Could you check a few things on this drawing? It's one solid part, dimensions in mm from its lowest x, y, z. A direction names the side the tool comes from. Give positions to 0.01 mm unless a question says otherwise; leave off trailing zeros. Order: outer loops, then holes, each group sorted by start corner. A loop starts at its lowest first (then second) coordinate and runs counter-clockwise, first axis right, second up.
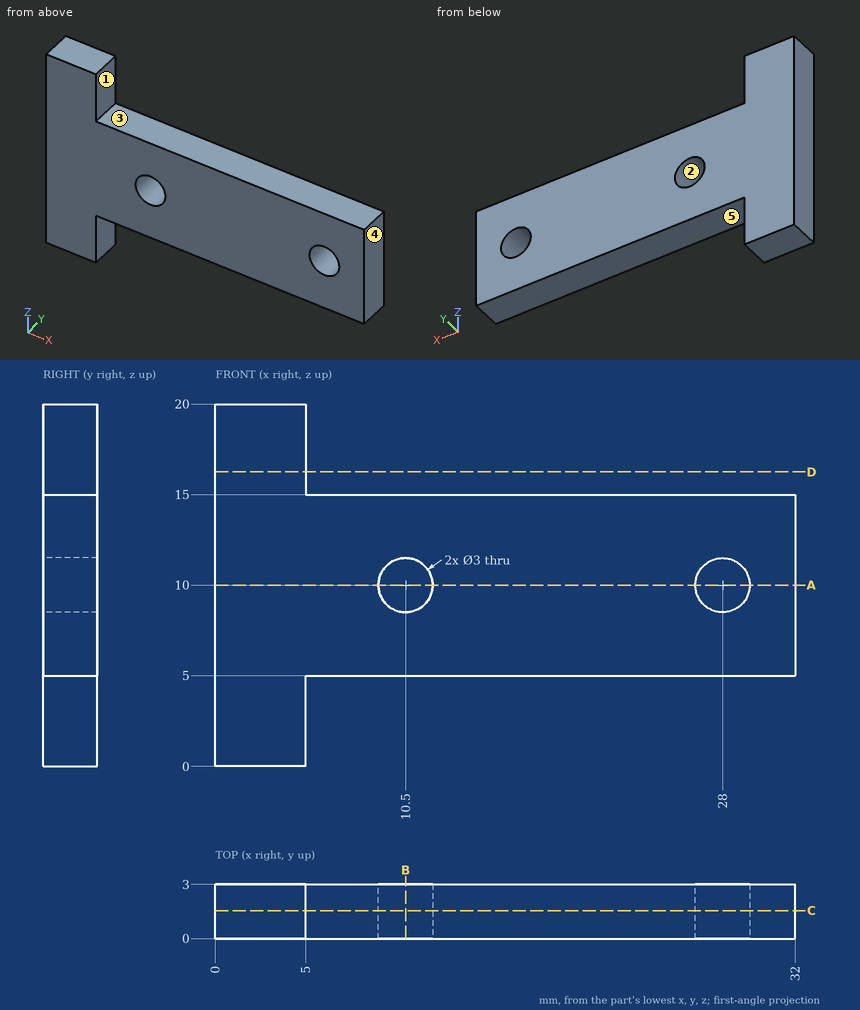
Q1. I'm going to push flat-ended pins straight in: P1, Ø1.5, axis at y = 1.5, z = 18.5, coming from the +X side; P2, Ø1.5, axis at x = 20, y = 1.5, coming from the -Z side. Where does each tip first touch, or does it pass through?
Filled sheet:
P1: stops at x = 5
P2: stops at z = 5
Q2. I need wall thicknesses on L1, parallel to Z at x = 28, y = 2.1; L2, parallel to Z at x = 25.5, y = 1.05; L3, parallel to X at y = 1.4, z = 9.75. Which ranges of each line are inside material? Lowest first, please.
Filled sheet:
L1: z = 5 to 8.5, 11.5 to 15
L2: z = 5 to 15
L3: x = 0 to 9.02, 11.98 to 26.52, 29.48 to 32
Q3. If we section it at C-C on y = 1.55: List the corners of the cut face in (x, z) for me, plus the area to 3 significant figures.
Filled sheet:
outline: (0, 0) - (5, 0) - (5, 5) - (32, 5) - (32, 15) - (5, 15) - (5, 20) - (0, 20) - close; hole circle Ø3 at (10.5, 10); hole circle Ø3 at (28, 10)
area: 356 mm2
Q4. If we section it at B-B on x = 10.5: List the corners of the cut face in (y, z) for me.
Filled sheet:
outline: (0, 5) - (3, 5) - (3, 8.5) - (0, 8.5) - close; (0, 11.5) - (3, 11.5) - (3, 15) - (0, 15) - close
Q5. If we section it at A-A on z = 10: List the corners of the cut face in (x, y) for me.
Filled sheet:
outline: (0, 0) - (9, 0) - (9, 3) - (0, 3) - close; (12, 0) - (26.5, 0) - (26.5, 3) - (12, 3) - close; (29.5, 0) - (32, 0) - (32, 3) - (29.5, 3) - close
Q6. Thinking about a two-plate mould opening in X: for the marked faces 1, 2 and 3, which applies, released by +X, released by -X, zero draft, split by the parting line, or undercut?
Filled sheet:
face 1: released by +X
face 2: undercut
face 3: zero draft
Q7. If we section it at D-D on z = 16.25: List the corners of the cut face in (x, y) for me, plus the area to 3 significant figures.
Filled sheet:
outline: (0, 0) - (5, 0) - (5, 3) - (0, 3) - close
area: 15.0 mm2
Q8. For the marked faces 4 and 5, which set-ups out of +Z, -Z, +X, -X, +Y, -Y let a thin tool reach every point of the face, with its end or its side?
Filled sheet:
face 4: +Z, -Z, +X, +Y, -Y
face 5: -Z, +X, +Y, -Y
